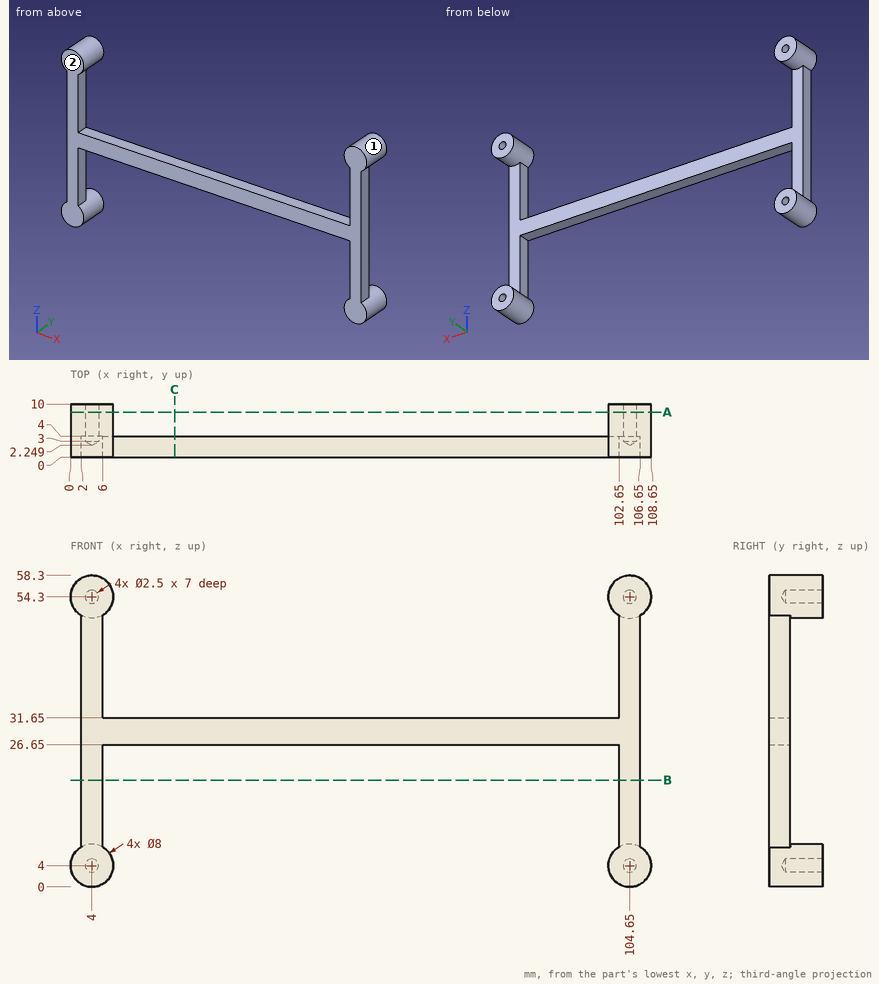
Part print with two shaded views. Sizes in mm from the minimum x, y, z corner. Give positions to 0.01 mm unless a question says otherwise; leave off trailing zeros. Order: outer loops, then holes, each group sorted by start corner. A loop starts at its lowest first (then second) coordinate and runs counter-clockwise, first axis right, second up.
(1) Mould opens along X. For the marked faces 1 and 2 say: released by +X, released by -X, zero draft, split by the parting line, or undercut.
(2) Saw through at C-C, the plane x = 19.5. Give the cut face in (y, z).
(3) Saw through at A-A, the plane y = 8.5. Give the cut face in (x, z), then the cut area to 3 significant figures.
(4) Saw through at B-B, the plane z = 20. Give the cut face in (x, y).
(5) Drill centre lines: L1, parallel to X at y = 6, z = 54.3; L2, parallel to Z at x = 104.65, y = 8; L3, parallel to Y at x = 68, z = 30.5. Where is each one in solid material? Low to high.
(6) Flat gauge pins, fed straight in: pin 1 (2 mm diameter, centred on x = 104.65, z = 4, fed in from +Y); pin 2 (1.2 mm diameter, centred on y = 1.5, z = 42.5, fed in from +X); pin 3 (5 mm diameter, centred on x = 56.5, y = 2.5, fed in from +Z). Where does each tip first touch, or does it go through?
Results found:
1. face 1: undercut
1. face 2: zero draft
2. outline: (0, 26.65) - (4, 26.65) - (4, 31.65) - (0, 31.65) - close
3. outline: circle Ø8 at (4, 4); circle Ø8 at (4, 54.3); circle Ø8 at (104.65, 4); circle Ø8 at (104.65, 54.3); hole circle Ø2.5 at (4, 4); hole circle Ø2.5 at (4, 54.3); hole circle Ø2.5 at (104.65, 4); hole circle Ø2.5 at (104.65, 54.3)
3. area: 181 mm2
4. outline: (2, 0) - (6, 0) - (6, 4) - (2, 4) - close; (102.65, 0) - (106.65, 0) - (106.65, 4) - (102.65, 4) - close
5. L1: x = 0 to 2.75, 5.25 to 8, 100.65 to 103.4, 105.9 to 108.65
5. L2: z = 0 to 2.75, 5.25 to 8, 50.3 to 53.05, 55.55 to 58.3
5. L3: y = 0 to 4
6. pin 1: stops at y = 2.85
6. pin 2: stops at x = 106.65
6. pin 3: stops at z = 31.65
